from build123d import *

# Parameters (mm, degrees)
F0_R     = 1.5
F1_DEPTH = 2


with BuildPart() as f1:
    # F0 (on Top) → F1 (new body)
    with BuildSketch(Plane.XY):
        with BuildLine():
            Line((-49.651527, 3.75), (-52.651527, 3.75))
            ThreePointArc((-52.651527, 3.75), (-54.772848, 2.87132), (-55.651527, 0.75))
            Line((-55.651527, 0.75), (-55.651527, -2.25))
            Line((-55.651527, -2.25), (-55.651527, -55.25))
            Line((-55.651527, -55.25), (-55.651527, -58.25))
            ThreePointArc((-55.651527, -58.25), (-54.772848, -60.37132), (-52.651527, -61.25))
            Line((-52.651527, -61.25), (-49.651527, -61.25))
            Line((-49.651527, -61.25), (38.348473, -61.25))
            Line((38.348473, -61.25), (41.348473, -61.25))
            ThreePointArc((41.348473, -61.25), (43.469793, -60.37132), (44.348473, -58.25))
            Line((44.348473, -58.25), (44.348473, -55.25))
            Line((44.348473, -55.25), (44.348473, -2.25))
            Line((44.348473, -2.25), (44.348473, 0.75))
            ThreePointArc((44.348473, 0.75), (43.469793, 2.87132), (41.348473, 3.75))
            Line((41.348473, 3.75), (38.348473, 3.75))
            Line((38.348473, 3.75), (-49.651527, 3.75))
        make_face()
        with Locations((-51.901527, -58.5)):
            Circle(F0_R, mode=Mode.SUBTRACT)
        with BuildLine():
            ThreePointArc((-34.449054, -58.25), (-37.332009, -56.079801), (-36.043907, -52.709047))
            Line((-36.043907, -52.709047), (-7.246381, -34.634004))
            ThreePointArc((-7.246381, -34.634004), (-5.651527, -34.174957), (-4.056674, -34.634004))
            Line((-4.056674, -34.634004), (24.740853, -52.709047))
            ThreePointArc((24.740853, -52.709047), (26.028954, -56.079801), (23.145999, -58.25))
            Line((23.145999, -58.25), (-34.449054, -58.25))
        make_face(mode=Mode.SUBTRACT)
        with Locations((40.098473, -58.5)):
            Circle(F0_R, mode=Mode.SUBTRACT)
        with BuildLine():
            ThreePointArc((-52.651527, -9.557936), (-51.103326, -6.93262), (-48.056674, -7.016983))
            Line((-48.056674, -7.016983), (-17.479486, -26.209047))
            ThreePointArc((-17.479486, -26.209047), (-16.07434, -28.75), (-17.479486, -31.290953))
            Line((-17.479486, -31.290953), (-48.056674, -50.483017))
            ThreePointArc((-48.056674, -50.483017), (-51.103326, -50.56738), (-52.651527, -47.942064))
            Line((-52.651527, -47.942064), (-52.651527, -9.557936))
        make_face(mode=Mode.SUBTRACT)
        with Locations((-51.901527, 0)):
            Circle(F0_R, mode=Mode.SUBTRACT)
        with BuildLine():
            Line((36.753619, -50.483017), (6.176432, -31.290953))
            ThreePointArc((6.176432, -31.290953), (4.771285, -28.75), (6.176432, -26.209047))
            Line((6.176432, -26.209047), (36.753619, -7.016983))
            ThreePointArc((36.753619, -7.016983), (39.800272, -6.93262), (41.348473, -9.557936))
            Line((41.348473, -9.557936), (41.348473, -47.942064))
            ThreePointArc((41.348473, -47.942064), (39.800272, -50.56738), (36.753619, -50.483017))
        make_face(mode=Mode.SUBTRACT)
        with BuildLine():
            Line((-7.246381, -22.865996), (-36.043907, -4.790953))
            ThreePointArc((-36.043907, -4.790953), (-37.332009, -1.420199), (-34.449054, 0.75))
            Line((-34.449054, 0.75), (23.145999, 0.75))
            ThreePointArc((23.145999, 0.75), (26.028954, -1.420199), (24.740853, -4.790953))
            Line((24.740853, -4.790953), (-4.056674, -22.865996))
            ThreePointArc((-4.056674, -22.865996), (-5.651527, -23.325043), (-7.246381, -22.865996))
        make_face(mode=Mode.SUBTRACT)
        with Locations((40.098473, 0)):
            Circle(F0_R, mode=Mode.SUBTRACT)
    extrude(amount=F1_DEPTH)


solid = f1.part
Read the model definition and answer for the solid it produces. Units are mm, in the model's axes. A direction names the side the tool comes from. Give positions to 0.01 mm unless a question says otherwise; leave off trailing zeros. Write each loop counter-clockwise with the first axis right and the second up, starting at its lowest first coordinate (ties: lowest second). Pieces come first, ordered by that corner, then holes. Notation, with made-up numbers: (-19.75, -4) -> (8.25, -4) arc R32 ccw to (8.25, 30) -> close; hole circle Ø3 at (-15.75, -5). An arc over 180 degrees is marked (long way). Answer as a JSON object with one key per item and string values. Group by question number.
1) A tool of negligible diameter and unlimited length cuts with its end or side. For faces 1 (the cylindrical face through (43.45, -60.39, 0.99)), 2 (the cylindrical face through (-37.317, -56.132, 0.986)), from which of +Z, -Z, +X, -X, +Y, -Y can it reach the whole face along a straight path? Write none if from no direction.
2) The mould has two halves that part along Y. Classify faces 3 (the cylindrical face through (26.013, -1.368, 0.986)), 4 (the flat face through (-6, -61.25, 1)), 5 (the cylindrical face through (43.49, 2.85, 0.99)): +Y half, -Y half, draft (parallel to the pull), parting line (faces both ways), or undercut.
3) Find section C-C (z = 0.75). Count the separate pieces of the cut face and the enclosed holes in it, and give its area (3 significant figures).
4) Consider L1, parallel to Y at x = -5.5, z = 1; L2, parallel to X at y = -55.5, z = 0.9; L3, parallel to X at y = -11, z = 1.65. Determine where each line is inside the solid, lowest interval first. Write a range as from..to.
5) Find section A-A (x = -38.5). Write down the section's boundary in (y, z).
6) Find section B-B (x = -23). Write down the section's boundary in (y, z).
7) Find section D-D (x = 30). Write down the section's boundary in (y, z), and give its area (3 significant figures).
Values follow:
{
 "1": {"face 1": "+Z, -Z, +X, -Y", "face 2": "+Z, -Z"},
 "2": {"face 3": "undercut", "face 4": "-Y half", "face 5": "+Y half"},
 "3": {"separate pieces": "1", "enclosed holes": "8", "area": "2,720 mm2"},
 "4": {"L1": "y = -61.25..-58.25, -34.18..-23.32, 0.75..3.75", "L2": "x = -55.65..-37.44, 26.14..44.35", "L3": "x = -55.65..-52.65, -41.71..-26.15, 14.85..30.41, 41.35..44.35"},
 "5": {"outline": "(-61.25, 0) -> (-44.48, 0) -> (-44.48, 2) -> (-61.25, 2) -> close; (-13.02, 0) -> (3.75, 0) -> (3.75, 2) -> (-13.02, 2) -> close"},
 "6": {"outline": "(-61.25, 0) -> (-58.25, 0) -> (-58.25, 2) -> (-61.25, 2) -> close; (-44.52, 0) -> (-34.76, 0) -> (-34.76, 2) -> (-44.52, 2) -> close; (-22.74, 0) -> (-12.98, 0) -> (-12.98, 2) -> (-22.74, 2) -> close; (0.75, 0) -> (3.75, 0) -> (3.75, 2) -> (0.75, 2) -> close"},
 "7": {"outline": "(-61.25, 0) -> (-46.24, 0) -> (-46.24, 2) -> (-61.25, 2) -> close; (-11.26, 0) -> (3.75, 0) -> (3.75, 2) -> (-11.26, 2) -> close", "area": "60.0 mm2"}
}
